Geometry check sheet. Reference: the model listing, model coordinates, mm. Give positions to 0.01 mm unless a question says otherwise; leave off trailing zeros. Order: outer loops, then holes, each group sorted by start corner. A loop starts at its lowest first (then second) coordinate and runs counter-clockwise, first axis right, second up. Notation, with made-up numbers: M -36.5,-0.5 L -31.5,-0.5 A11 ccw -31.5,9.5 Z; hole C 15.5,62.25 d6. An arc over 180 degrees is marked long. One line per question, with ' | ' between items. Start each with the question number.
from build123d import *

# Parameters (mm, degrees)
EXTRUDE_1_DEPTH = 200


# Read off the part's stored shape, not the designer's step: 本體-刪除/保留 2, 本體-刪除/保留 3, 本體-刪除/保留 4
with BuildPart() as part:
    # 草圖1 → 填料-伸長1 (new body)
    with BuildSketch(Plane(origin=(0, 0, 0), x_dir=(1, 0, 0), z_dir=(0, 1, 0))):
        Polygon((0, 100), (-100, 0), (0, -100), (100, 0), align=None)
    extrude(amount=EXTRUDE_1_DEPTH)


with BuildPart() as body_2:
    # Split Bodies 2: the piece on the far side of the plane
    add(part.part)
    split(bisect_by=Plane(origin=(-44.444444444, 22.222222222, -44.444444444), x_dir=(0.7071067811865474, 0, -0.7071067811865479), z_dir=(-0.666666666666667, 0.33333333333333337, -0.6666666666666665)), keep=Keep.BOTTOM)


with BuildPart() as part_1:
    add(part.part)

    # Split Bodies 2
    split(bisect_by=Plane(origin=(-44.444444444, 22.222222222, -44.444444444), x_dir=(0.7071067811865474, 0, -0.7071067811865479), z_dir=(-0.666666666666667, 0.33333333333333337, -0.6666666666666665)), keep=Keep.TOP)


with BuildPart() as body_2_2:
    # Split Bodies 3: the piece on the far side of the plane
    add(body_2.part)
    split(bisect_by=Plane(origin=(-42.372881356, 25.423728814, 42.372881356), x_dir=(0.7071067811865476, 0, 0.7071067811865476), z_dir=(-0.6509445549041194, 0.39056673294247174, 0.6509445549041194)), keep=Keep.BOTTOM)


with BuildPart() as body_2_1:
    add(body_2.part)

    # Split Bodies 3
    split(bisect_by=Plane(origin=(-42.372881356, 25.423728814, 42.372881356), x_dir=(0.7071067811865476, 0, 0.7071067811865476), z_dir=(-0.6509445549041194, 0.39056673294247174, 0.6509445549041194)), keep=Keep.TOP)


with BuildPart() as body_2_3:
    # Split Bodies 4: the piece on the far side of the plane
    add(body_2_2.part)
    split(bisect_by=Plane(origin=(44.444444444, 22.222222222, 44.444444444), x_dir=(0.7071067811865479, 0, -0.7071067811865474), z_dir=(0.6666666666666665, 0.33333333333333337, 0.666666666666667)), keep=Keep.BOTTOM)


with BuildPart() as body_2_2_1:
    add(body_2_2.part)

    # Split Bodies 4
    split(bisect_by=Plane(origin=(44.444444444, 22.222222222, 44.444444444), x_dir=(0.7071067811865479, 0, -0.7071067811865474), z_dir=(0.6666666666666665, 0.33333333333333337, 0.666666666666667)), keep=Keep.TOP)


with BuildPart() as body_2_4:
    # Split Bodies 5: the piece on the far side of the plane
    add(body_2_3.part)
    split(bisect_by=Plane(origin=(46.296296296, 18.518518519, -46.296296296), x_dir=(-0.7071067811865475, 0, -0.7071067811865477), z_dir=(-0.6804138174397718, -0.2721655269759089, 0.6804138174397716)), keep=Keep.BOTTOM)


with BuildPart() as body_2_3_1:
    add(body_2_3.part)

    # Split Bodies 5
    split(bisect_by=Plane(origin=(46.296296296, 18.518518519, -46.296296296), x_dir=(-0.7071067811865475, 0, -0.7071067811865477), z_dir=(-0.6804138174397718, -0.2721655269759089, 0.6804138174397716)), keep=Keep.TOP)


solid = body_2_3_1.part
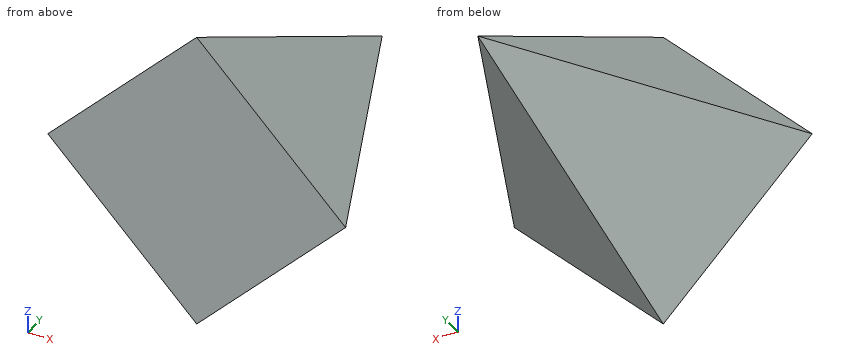
Item 1: Cross-section at D-D, the plane y = 134. Record the cut outline in (x, z), plus the area to 3 significant figures.
Item 2: Cross-section at B-B, the plane x = 55. Record the cut outline in (y, z), plus the area to 3 significant figures.
Item 3: Material ranges on line 1 along X through (y, z) = (87, 39); line 2 along Z through (x, y) = (86, 18.5); line 3 along Y through (x, z) = (-8, -20.5), recorded low to high.
Item 4: Depth check by flat-ended pin: pin 1 (3 mm diameter, centred on y = 24, z = 27.5, fed in from -X); pin 2 (3 mm diameter, centred on x = -56.5, y = 80.5, fed in from -Z); pin 3 (1.5 mm diameter, centred on y = 73, z = 13.5, fed in from +X). Enter the tip coordinate at first touch or a pass-through.
Item 5: Cross-section at C-C, the plane z = -54. Record the cut outline in (x, y), plus the area to 3 significant figures.
Item 6: Cross-section at A-A, the plane y = 26. Record the cut outline in (x, z).
Outcome:
1) outline: M -26.3,-6.7 L 6.7,-39.7 L 39.7,-6.7 L 6.7,26.3 Z | area: 2,180 mm²
2) outline: M 0,-45 L 100,-5 L 0,45 Z | area: 4,500 mm²
3) line 1: x = -8.8 to 17.5 | line 2: z = -6.6 to 4.75 | line 3: y = 0 to 143
4) pin 1: stops at x = -59.85 | pin 2: stops at z = -4.93 | pin 3: stops at x = 50.84
5) outline: M -46,0 L 46,0 L 5.11,102.22 Z | area: 4,700 mm²
6) outline: M -85.7,-1.3 L 1.3,-88.3 L 88.3,-1.3 L 1.3,85.7 Z
